```python
from build123d import *

# Parameters (mm, degrees)
BOSS_EXTRUDE1_DEPTH             = 1.905
F_3_0MM_DOWEL_HOLE1_D           = 3.2
F_3_0MM_DOWEL_HOLE1_CSINK_D     = 3.3
F_3_0MM_DOWEL_HOLE1_CSINK_ANGLE = 90


with BuildPart() as part:
    # Sketch1 → Boss-Extrude1 (new body)
    with BuildSketch(Plane.XY):
        with BuildLine():
            Line((-50.6, 15.04), (50.6, 15.04))
            Line((50.6, 15.04), (54.590317598, 7.813493896))
            ThreePointArc((54.590317598, 7.813493896), (56.604225159, 0), (54.590317598, -7.813493896))
            Line((54.590317598, -7.813493896), (50.6, -15.04))
            Line((50.6, -15.04), (-50.6, -15.04))
            Line((-50.6, -15.04), (-54.590317598, -7.813493896))
            ThreePointArc((-54.590317598, -7.813493896), (-56.604225159, 0), (-54.590317598, 7.813493896))
            Line((-54.590317598, 7.813493896), (-50.6, 15.04))
        make_face()
    extrude(amount=BOSS_EXTRUDE1_DEPTH)

    # Ø3.0mm Dowel Hole1 (through all)
    with Locations(Plane.XY.offset(1.905)):
        with Locations((53.975, 0), (-53.975, 0)):
            CounterSinkHole(F_3_0MM_DOWEL_HOLE1_D / 2, F_3_0MM_DOWEL_HOLE1_CSINK_D / 2, counter_sink_angle=F_3_0MM_DOWEL_HOLE1_CSINK_ANGLE)


solid = part.part
```
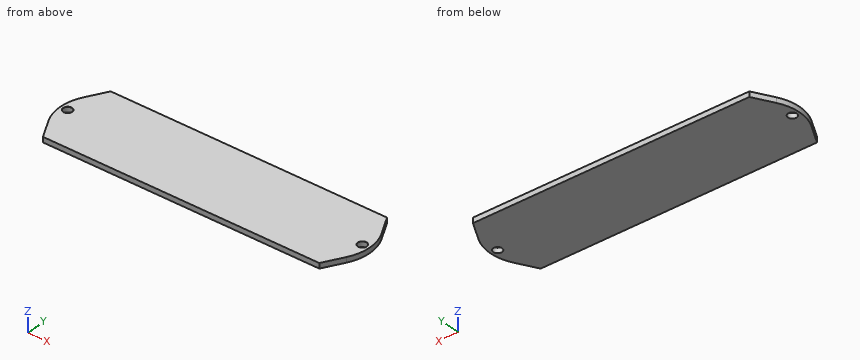
For this review, take the finished solid that the model builds, in its own axes (mm). Coordinates: 2 decimals unless noted, no trailing zeros. Loops run counter-clockwise (first coordinate to the right, second up) from the corner with the lowest first, then second, coordinate; pieces in that order, holes last.
1. Add section A-A, the plane z = 1.3. Give the boundary of the cut face in (x, y) (1 decimal), then the cut area to 3 significant figures.
2. Add section C-C, the plane y = -10. Give the boundary of the cut face in (x, z) (3 decimals), then the cut area to 3 significant figures.
3. Add section B-B, the plane y = 0. Give the boundary of the cut face in (x, z) (3 decimals).
4. Insertion check: P1, Ø1.5, axis at x = 2, y = 3, coming from the -Z side. The pin has a flat end and moves straight along its axis. Give the tip position at first contact, or say it passes through.
5. For line 1 (Y direction, x = -52, z = 1.6); line 2 (X direction, y = -2, z = 0.3); line 3 (X direction, y = 13, z = 1), list the stretches that pass through material, from the lowest coordinate up.
6. Add section D-D, the plane y = 12. Give the boundary of the cut face in (x, z) (3 decimals).
Result:
1. outline: (-54.6, -7.8) - (-50.6, -15) - (50.6, -15) - (54.6, -7.8) arc R16.2 ccw to (54.6, 7.8) - (50.6, 15) - (-50.6, 15) - (-54.6, 7.8) arc R16.2 ccw to start; hole circle Ø3.2 at (-54, 0); hole circle Ø3.2 at (54, 0)
1. area: 3,250 mm2
2. outline: (-53.383, 0) - (53.383, 0) - (53.383, 1.905) - (-53.383, 1.905) - close
2. area: 203 mm2
3. outline: (-56.604, 0) - (-55.575, 0) - (-55.575, 1.855) - (-55.625, 1.905) - (-56.604, 1.905) - close; (-52.375, 0) - (52.375, 0) - (52.375, 1.855) - (52.325, 1.905) - (-52.325, 1.905) - (-52.375, 1.855) - close; (55.575, 0) - (56.604, 0) - (56.604, 1.905) - (55.625, 1.905) - (55.575, 1.855) - close
4. P1: stops at z = 0
5. line 1: y = -12.5 to 12.5
5. line 2: x = -56.48 to 56.48
5. line 3: x = -51.73 to 51.73
6. outline: (-52.279, 0) - (52.279, 0) - (52.279, 1.905) - (-52.279, 1.905) - close
